Design review of the part built by this model. Coordinates are the model's own, in mm. Face numbers are marked on the shaded views. A direction names the side the tool comes from. Round coordinates to 2 decimals unless told otherwise and drop trailing zeros. Order: outer loops, then holes, each group sorted by start corner. A loop starts at its lowest first (then second) coordinate and runs counter-clockwise, first axis right, second up. Notation, with made-up numbers: M -27.75,-30.5 L 23.25,-30.5 A17 ccw 23.25,-1.5 Z; hole C 44,15.25 d5. An arc over 180 degrees is marked long. Write each question's results on one line, items separated by ' | '. Start each with the question number.
Item 1: Clearance check with flat-ended pins moving along their axes: pin 1 (5 mm diameter, centred on y = 8.5, z = 4.5, fed in from +X); pin 2 (1 mm diameter, centred on y = 0.5, z = 20.5, fed in from -X) (3 decimals); pin 3 (2 mm diameter, centred on x = 6.5, z = 21.5, fed in from -Y). State where each tip first meets the part, or that it passes through.
Item 2: Take a section at A-A, the plane z = 17.5. Write out the cut boundary in (x, y), plus the area to 3 significant figures.
Item 3: Take a section at B-B, the plane x = -1.5. Write out the cut boundary in (y, z), plus the area to 3 significant figures.
Item 4: Take a section at D-D, the plane z = 6.5. Write out the cut boundary in (x, y), plus the area to 3 significant figures.
Item 5: Take a section at C-C, the plane y = -4.5. Write out the cut boundary in (x, z).
Item 6: Wall thickness on line 1 (Z direction, x = 0.5, y = 6.75); line 2 (Z direction, x = 10.25, y = 6); line 3 (Y direction, x = -6.5, z = 19): over which ranges is each line inside the solid? List them lowest first. Write a range as [from, to].
Item 7: Machinability: for the marked faces 1, 2 and 3, which of the approach directions +Z, -Z, +X, -X, +Y, -Y give a long, thin tool a straight path to every point of the face, cutting with its end or side? Answer none if there is none.
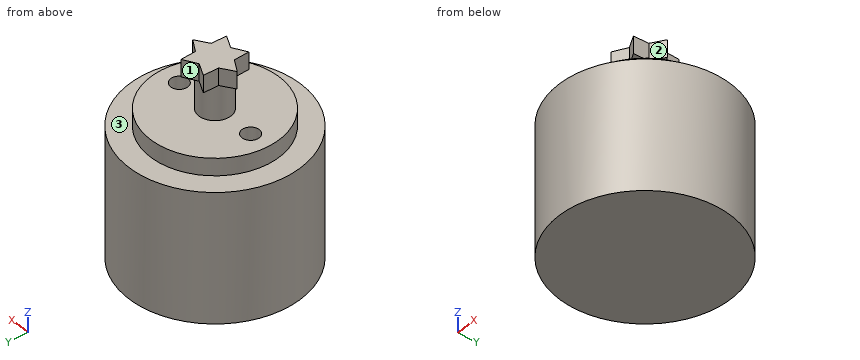
Autodesk Inventor part; units mm, degrees
ref_plane "Work Plane1" through (0, 0, 26.67) normal (0, 0, 1) x (1, 0, 0)
ref_plane "YZ Plane" through (0, 0, 0) normal (1, 0, 0) x (0, 1, 0)
ref_plane "XZ Plane" through (0, 0, 0) normal (0, 1, 0) x (-1, 0, 0)
sketch "Sketch1" plane through (0, 0, 0) normal (0, 0, 1) x (1, 0, 0)
  circle A0 centre (0, 0) radius 12.7
  dimension "d0" = 25.4
extrude "Extrusion1" add sketch "Sketch1" along normal blind 19.05
sketch "Sketch2" plane through (0, 0, 19.05) normal (0, 0, 1) x (1, 0, 0)
  circle A0 centre (0, 0) radius 9.525
  dimension "d3" = 19.05
extrude "Extrusion2" add sketch "Sketch2" along normal blind 1.27
sketch "Sketch3" plane through (0, 0, 20.32) normal (0, 0, 1) x (1, 0, 0)
  circle A0 centre (0, 0) radius 9.525
  dimension "d6" = 19.05
extrude "Extrusion3" add sketch "Sketch3" along normal blind 1.27
sketch "Sketch4" plane through (0, 0, 21.59) normal (0, 0, 1) x (1, 0, 0)
  circle A0 centre (0, 0) radius 2.3729
extrude "Extrusion4" add sketch "Sketch4" along normal blind 5.08
ref_plane "Work Plane1" through (0, 0, 26.67) normal (0, 0, 1) x (1, 0, 0)
sketch "Sketch10" plane through (0, 0, 26.67) normal (0, 0, 1) x (1, 0, 0)
  circle A0 centre (0, 0) radius 2.3813 construction
  circle A1 centre (0, 0) radius 3.9688 construction
  line L0 (0, 4.2939) -> (0, -5.5705) construction
  line L1 (6.3712, 0) -> (-7.3964, 0) construction
  line L2 (0, 2.3813) -> (1.9844, 3.437)
  line L3 (1.9844, 3.437) -> (2.0622, 1.1906)
  line L4 (-2.0622, 1.1906) -> (-1.9844, 3.437)
  line L5 (-1.9844, 3.437) -> (0, 2.3813)
  line L6 (-2.0622, -1.1906) -> (-3.9688, 0)
  line L7 (-3.9688, 0) -> (-2.0622, 1.1906)
  line L8 (0, -2.3813) -> (-1.9844, -3.437)
  line L9 (-1.9844, -3.437) -> (-2.0622, -1.1906)
  line L10 (2.0622, -1.1906) -> (1.9844, -3.437)
  line L11 (1.9844, -3.437) -> (0, -2.3813)
  line L12 (2.0622, 1.1906) -> (3.9688, 0)
  line L13 (3.9688, 0) -> (2.0622, -1.1906)
  line L14 (-2.0622, -1.1906) -> (0, -2.3813)
  line L15 (0, -2.3813) -> (2.0622, -1.1906)
  line L16 (2.0622, -1.1906) -> (2.0622, 1.1906)
  line L17 (2.0622, 1.1906) -> (0, 2.3813)
  line L18 (0, 2.3813) -> (-2.0622, 1.1906)
  line L19 (-2.0622, 1.1906) -> (-2.0622, -1.1906)
  line L20 (-2.0622, 1.1906) -> (0, 2.3813)
  line L21 (2.0622, 1.1906) -> (0, 2.3813)
  line L22 (2.0622, 1.1906) -> (2.0622, -1.1906)
  line L23 (2.0622, -1.1906) -> (0, -2.3813)
  line L24 (0, -2.3813) -> (-2.0622, -1.1906)
  line L25 (-2.0622, -1.1906) -> (-2.0622, 1.1906)
  line L26 (-3.9688, 0) -> (-2.0622, 1.1906)
  line L27 (-2.0622, -1.1906) -> (-2.0622, 1.1906)
  line L28 (-2.0622, -1.1906) -> (-3.9688, 0)
  line L29 (0, -2.3813) -> (-1.9844, -3.437)
  line L30 (-1.9844, -3.437) -> (-2.0622, -1.1906)
  line L31 (-2.0622, -1.1906) -> (0, -2.3812)
  line L32 (2.0622, -1.1906) -> (1.9844, -3.437)
  line L33 (1.9844, -3.437) -> (0, -2.3813)
  line L34 (0, -2.3812) -> (2.0622, -1.1906)
  line L35 (2.0622, 1.1906) -> (3.9688, 0)
  line L36 (3.9688, 0) -> (2.0622, -1.1906)
  line L37 (2.0622, -1.1906) -> (2.0622, 1.1906)
  line L38 (0, 2.3813) -> (1.9844, 3.437)
  line L39 (1.9844, 3.437) -> (2.0622, 1.1906)
  line L40 (2.0622, 1.1906) -> (0, 2.3813)
  line L41 (-2.0622, 1.1906) -> (-1.9844, 3.437)
  line L42 (-1.9844, 3.437) -> (0, 2.3813)
  line L43 (0, 2.3813) -> (-2.0622, 1.1906)
  line L44 (-2.0622, 1.1906) -> (0, 2.3813)
  line L45 (0, 2.3813) -> (-1.9844, 3.437)
  line L46 (-1.9844, 3.437) -> (-2.0622, 1.1906)
  line L47 (0, 2.3813) -> (1.9844, 3.437)
  line L48 (1.9844, 3.437) -> (2.0622, 1.1906)
  line L49 (0, 2.3813) -> (2.0622, 1.1906)
  line L50 (2.0622, 1.1906) -> (2.0622, -1.1906)
  line L51 (2.0622, -1.1906) -> (3.9688, 0)
  line L52 (3.9688, 0) -> (2.0622, 1.1906)
  line L53 (2.0622, -1.1906) -> (0, -2.3812)
  line L54 (0, -2.3812) -> (1.9844, -3.437)
  line L55 (1.9844, -3.437) -> (2.0622, -1.1906)
  line L56 (0, -2.3812) -> (-1.9844, -3.437)
  line L57 (-2.0622, -1.1906) -> (-1.9844, -3.437)
  line L58 (-2.0622, -1.1906) -> (0, -2.3812)
  line L59 (-2.0622, -1.1906) -> (-2.0622, 1.1906)
  line L60 (-2.0622, 1.1906) -> (-3.9688, 0)
  line L61 (-3.9688, 0) -> (-2.0622, -1.1906)
  point P0 (3.9688, 0)
  point P1 (-1.9844, 3.437)
  point P2 (-3.9688, 0)
  point P3 (-1.9844, -3.437)
  point P4 (1.9844, -3.437)
  dimension "d26" = 4.7625
  dimension "d27" = 7.9375
  dimension "d30" = 360
  dimension "d34" = 360
  dimension "d38" = 360
  dimension "d42" = 360
extrude "Extrusion10" add sketch "Sketch10" along normal blind 2.54
sketch "Sketch11" plane through (0, 0, 21.59) normal (0, 0, 1) x (1, 0, 0)
  point P0 (0, 0)
  point P1 (-6.35, 0)
  point P2 (6.35, 0)
  dimension "d46" = 6.35
  dimension "d47" = 6.35
hole "Hole1" at (-6.35, 0, 21.59) at (6.35, 0, 21.59) direction (0, 0, -1) diameter 2.54 depth 12.7 tip angle 118
properties part number "000109"
Results list:
1) pin 1: x = 11.19 | pin 2: x = -9.525 | pin 3: y = -7.78
2) outline: C 0,0 d25.4; hole C -6.35,0 d2.54; hole C 6.35,0 d2.54 | area: 497 mm²
3) outline: M -12.61,0 L 12.61,0 L 12.61,19.05 L 9.41,19.05 L 9.41,21.59 L 1.84,21.59 L 1.84,26.67 L 3.18,26.67 L 3.18,29.21 L -3.18,29.21 L -3.18,26.67 L -1.84,26.67 L -1.84,21.59 L -9.41,21.59 L -9.41,19.05 L -12.61,19.05 Z | area: 563 mm²
4) outline: C 0,0 d25.4 | area: 507 mm²
5) outline: M -11.88,0 L 11.88,0 L 11.88,19.05 L 8.39,19.05 L 8.39,21.59 L -8.39,21.59 L -8.39,19.05 L -11.88,19.05 Z
6) line 1: [0, 21.59] | line 2: [0, 19.05] | line 3: [-10.91, -1.26], [1.26, 10.91]
7) face 1: +Z, +Y | face 2: +Z, +X, -Y | face 3: +Z
